Job drawing, mm, ordinate dimensions from the low corner. One solid piece. Coordinates: 2 decimals unless noted, no trailing zeros. Order: outer loops, then holes, each group sorted by start corner. A loop starts at its lowest first (then second) coordinate and runs counter-clockwise, first axis right, second up. Notation, with made-up numbers: M -23.75,14.5 L 22.25,14.5 A26 ccw 22.25,28.5 Z; hole C 9,77 d7. An arc over 180 degrees is marked long. Write item = value, one per line. Start each with the question number.
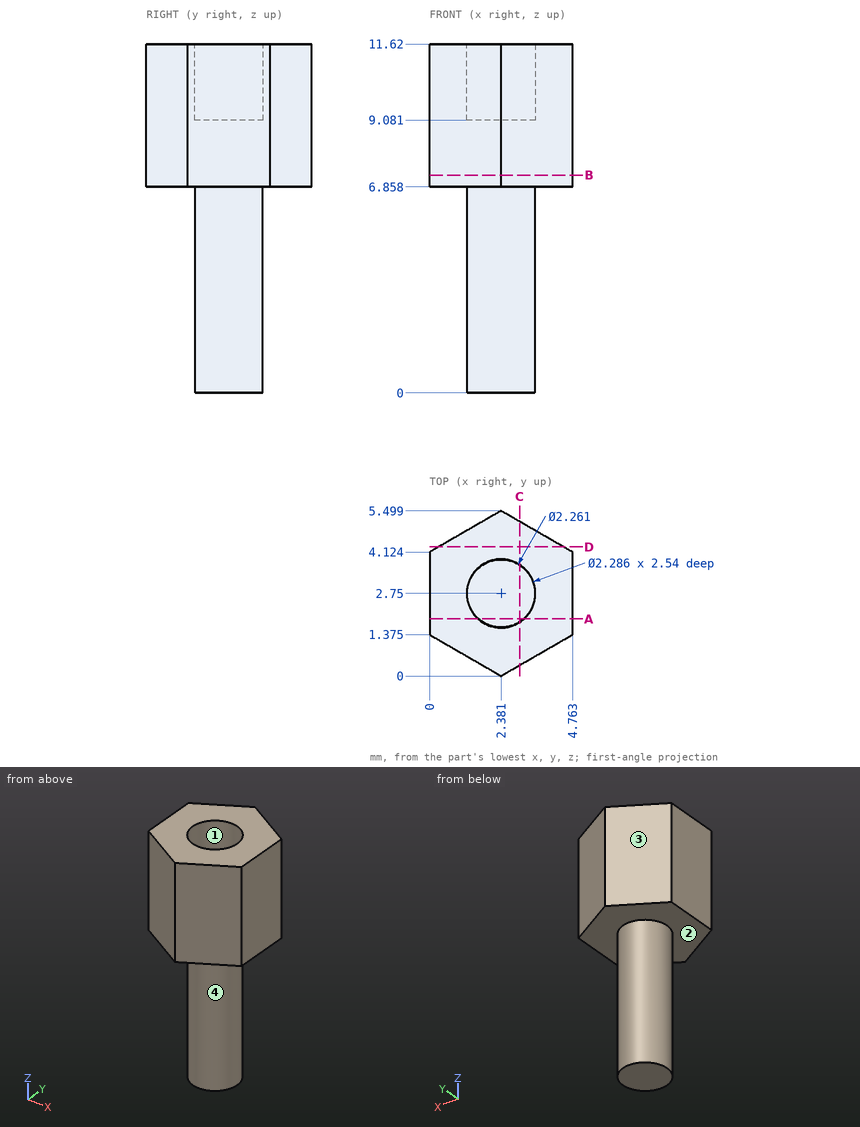
1. Flat gauge pins, fed straight in: pin 1 (2 mm diameter, centred on x = 3, z = 4.5, fed in from -Y); pin 2 (2 mm diameter, centred on x = 2, z = 4, fed in from +Y). Where does each tip first touch, or does it go through?
2. Mould opens along X. For the marked faces 1, 2, 3 and 4 say: released by +X, released by -X, zero draft, split by the parting line, or undercut.
3. Slice it at C-C (x = 3). Write the cut outline in (y, z) (1 decimal).
4. Slice it at A-A (y = 1.9). Write the cut outline in (x, z) (1 decimal).
5. Slice it at D-D (y = 4.3). Write the cut outline in (x, z) (1 decimal), plus the area to 3 significant figures.
6. Probe L1, parallel to Z at x = 3.95, y = 2.3; L2, parallel to X at y = 2.3, z = 9.5; L3, parallel to Y at x = 2.95, z = 11.25. List the from-to ranges inside material, lowest first.
7. Slice it at B-B (z = 7.25). Write the cut outline in (x, y) (1 decimal).
Calculated:
q1.pin_1 = 1.62
q1.pin_2 = 3.88
q2.face_1 = undercut
q2.face_2 = zero draft
q2.face_3 = released by -X
q2.face_4 = split by the parting line
q3.outline = M 0.4,6.9 L 1.8,6.9 L 1.8,0 L 3.7,0 L 3.7,6.9 L 5.1,6.9 L 5.1,11.6 L 3.7,11.6 L 3.7,9.1 L 1.8,9.1 L 1.8,11.6 L 0.4,11.6 Z
q4.outline = M 0,6.9 L 1.6,6.9 L 1.6,0 L 3.1,0 L 3.1,6.9 L 4.8,6.9 L 4.8,11.6 L 3.1,11.6 L 3.1,9.1 L 1.6,9.1 L 1.6,11.6 L 0,11.6 Z
q5.outline = M 0.3,6.9 L 4.5,6.9 L 4.5,11.6 L 0.3,11.6 Z
q5.area = 19.8 mm²
q6.L1 = 6.86 to 11.62
q6.L2 = 0 to 1.33, 3.43 to 4.76
q6.L3 = 0.33 to 1.76, 3.74 to 5.17
q7.outline = M 0,1.4 L 2.4,0 L 4.8,1.4 L 4.8,4.1 L 2.4,5.5 L 0,4.1 Z
